```python
from build123d import *

# Parameters (mm, degrees)
SKETCH1_R               = 4.4
BOSS_EXTRUDE1_DEPTH     = 8.8
SKETCH2_R               = 4.737731287
SKETCH2_R_2             = 4
BOSS_EXTRUDE2_DEPTH     = 6.25
CUT_EXTRUDE1_DEPTH      = 12.787646148
CUT_EXTRUDE1_DEPTH_BACK = 12.787646148
SKETCH3_R               = 4


with BuildPart() as part:
    # Sketch1 → Boss-Extrude1 (new body)
    with BuildSketch(Plane.YZ):
        with Locations(Location((0, 0, 0), (0, 0, 270))):
            Circle(SKETCH1_R)
    extrude(amount=BOSS_EXTRUDE1_DEPTH)

    # Sketch2 → Boss-Extrude2 (add, symmetric)
    with BuildSketch(Plane(origin=(0, 0, 0), x_dir=(-1, 0, 0), z_dir=(0, 1, 0))):
        with Locations(Location((0, 0, 0), (0, 0, 90))):
            Circle(SKETCH2_R)
        with Locations(Location((0, 0, 0), (0, 0, 90))):
            Circle(SKETCH2_R_2, mode=Mode.SUBTRACT)
    extrude(amount=BOSS_EXTRUDE2_DEPTH, both=True)

    # Sketch3 → Cut-Extrude1 (cut, two sides: drawn at the far end of the back side and taken through both)
    with BuildSketch(Plane(origin=(0, 0, 0), x_dir=(-1, 0, 0), z_dir=(0, 1, 0)).offset(-CUT_EXTRUDE1_DEPTH_BACK)):
        with Locations(Location((0, 0, 0), (0, 0, 90))):
            Circle(SKETCH3_R)
    extrude(amount=CUT_EXTRUDE1_DEPTH + CUT_EXTRUDE1_DEPTH_BACK, mode=Mode.SUBTRACT)


solid = part.part
```
CAD build for the part. Positions are in the model's coordinates, mm. A direction names the side the tool comes from. Coordinates: 2 decimals unless noted, no trailing zeros. Order: outer loops, then holes, each group sorted by start corner. A loop starts at its lowest first (then second) coordinate and runs counter-clockwise, first axis right, second up. Notation, with made-up numbers: (-15.5, 24.25) -> (12.5, 24.25) arc R32 ccw to (12.5, 61.25) -> close; hole circle Ø2 at (66.25, 21.5). An arc over 180 degrees is marked (long way). Use one line per item in the form item = value. Start each with the question number.
1) Band-saw the part on B-B on z = 0. Give the cut face in (x, y), then the cut area to 3 significant figures.
2) Drop flat-ended pins along their axis: pin 1 (3 mm diameter, centred on x = -0.5, z = -1.5, fed in from +Y); pin 2 (2 mm diameter, centred on x = -1.5, y = 0.5, fed in from +Z); pin 3 (1.5 mm diameter, centred on x = 6, y = 3, fed in from +Z); pin 4 (1.5 mm diameter, centred on x = 5.5, y = 3, fed in from -Z). Give the stop position or say it passes through.
3) Band-saw the part on C-C on y = 0. Give the cut face in (x, z).
4) Tool access for faces 1 (the cylindrical face through (6.012, 0.193, 4.396)), 2 (the flat face through (-2, -6.25, -4)): list every direction of +Z, -Z, +X, -X, +Y, -Y with a clear straight run to the whole face (end or side of a thin tool).
5) Pull direction X, two halves, no side cores. Call faces 3 (the cylindrical face through (-4.625, 0.088, -1.027)), 4 (the flat face through (8.8, 0, 0)), 5 (the cylindrical face through (-3.905, -0.088, -0.867)): +X half, -X half, draft (parallel to the pull), parting line (faces both ways), or undercut.
6) Drill centre lines: L1, parallel to X at y = 1.75, z = 0; L2, parallel to X at y = 0.5, z = -1.25; L3, parallel to Z at x = -2, y = 1.75. Where is each one in solid material? Low to high. Write a range as [from, to].
7) Band-saw the part on A-A on x = 0. Give the cut face in (y, z).
8) Band-saw the part on D-D on z = -2.25. Give the cut face in (x, y), then the cut area to 3 significant figures.
Entries:
q1.outline = (-4.74, -6.25) -> (-4, -6.25) -> (-4, 6.25) -> (-4.74, 6.25) -> close; (4, -6.25) -> (4.74, -6.25) -> (4.74, -4.4) -> (8.8, -4.4) -> (8.8, 4.4) -> (4.74, 4.4) -> (4.74, 6.25) -> (4, 6.25) -> close
q1.area = 54.2 mm2
q2.pin_1 = through
q2.pin_2 = 4.71
q2.pin_3 = 3.78
q2.pin_4 = -3.78
q3.outline = (1.76, -4.4) -> (8.8, -4.4) -> (8.8, 4.4) -> (1.76, 4.4) arc R4.74 ccw (long way) to start; hole circle Ø8 at (0, 0)
q4.face_1 = +X
q4.face_2 = +Z, -Z, +X, -X, -Y
q5.face_3 = parting line
q5.face_4 = +X half
q5.face_5 = undercut
q6.L1 = [-4.74, -4], [4, 8.8]
q6.L2 = [-4.57, -3.8], [3.8, 8.8]
q6.L3 = [-4.29, -3.46], [3.46, 4.29]
q7.outline = (-6.25, -4.74) -> (6.25, -4.74) -> (6.25, -4) -> (-6.25, -4) -> close; (-6.25, 4) -> (6.25, 4) -> (6.25, 4.74) -> (-6.25, 4.74) -> close
q8.outline = (-4.17, -6.25) -> (-3.31, -6.25) -> (-3.31, 6.25) -> (-4.17, 6.25) -> close; (3.31, -6.25) -> (4.17, -6.25) -> (4.17, -3.78) -> (8.8, -3.78) -> (8.8, 3.78) -> (4.17, 3.78) -> (4.17, 6.25) -> (3.31, 6.25) -> close
q8.area = 56.6 mm2
